```python
from build123d import *

# Parameters (mm, degrees)
CUT_EXTRUDE4_DEPTH      = 10.5250001
CUT_EXTRUDE4_DEPTH_BACK = 10.5250001
CHAMFER1_SIZE           = 0.762


with BuildPart() as part:
    # Sketch1 → Revolve1 (revolve)
    with BuildSketch(Plane(origin=(0, 0, 0), x_dir=(0, 0, -1), z_dir=(1, 0, 0))):
        with BuildLine():
            Line((0, 0), (3.175, 0))
            Line((3.175, 0), (3.175, 9.4996))
            Line((3.175, 9.4996), (9.525, 9.4996))
            Line((9.525, 9.4996), (9.525, 12.7))
            ThreePointArc((9.525, 12.7), (4.820045897, 13.835459863), (0, 14.2748))
            Line((0, 14.2748), (0, 0))
        make_face()
    revolve(axis=Axis((0, 0, 0), (0, 1, 0)))

    # Sketch2 → Cut-Extrude4 (cut, two sides)
    with BuildSketch(Plane(origin=(0, 0, 0), x_dir=(0, 0, -1), z_dir=(1, 0, 0))) as cut_extrude4_sk:
        Polygon((-0.7874, 59.433466129), (-0.7874, 14.251322907), (-0.7874, 11.8872), (0.7874, 11.8872), (0.7874, 14.251322907), (0.7874, 59.433466129), (0.7874, 149.797752573), (-0.7874, 149.797752573), align=None)
    extrude(amount=CUT_EXTRUDE4_DEPTH, mode=Mode.SUBTRACT)
    extrude(cut_extrude4_sk.sketch, amount=-CUT_EXTRUDE4_DEPTH_BACK, mode=Mode.SUBTRACT)

    # Chamfer1
    chamfer1_edges = [part.edges().sort_by_distance(p)[0] for p in [
        (0, 0, 3.175),
    ]]
    chamfer(chamfer1_edges, length=CHAMFER1_SIZE)


solid = part.part
```
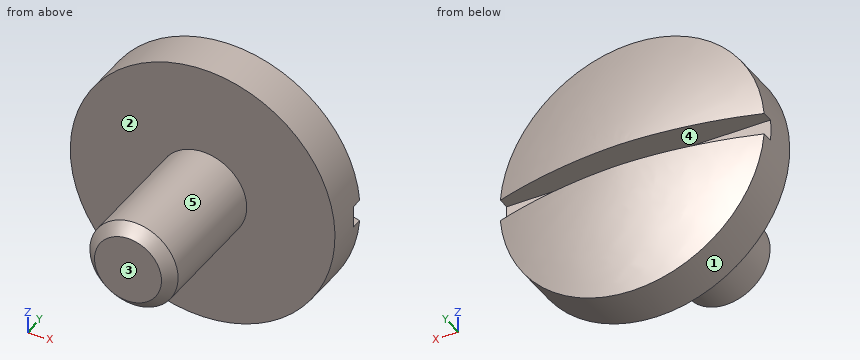
Source: CAD feature listing. Evaluate the final solid. Frame: model axes, mm. Face numbers are marked on the shaded views. A direction names the side the tool comes from. Coordinates: 2 decimals unless noted, no trailing zeros. Write each loop counter-clockwise with the first axis right and the second up, starting at its lowest first coordinate (ties: lowest second). Pieces come first, ordered by that corner, then holes. Notation, with made-up numbers: (34, 59) -> (85, 59) arc R19 ccw to (85, 65) -> close; hole circle Ø3 at (64, 26). An arc over 180 degrees is marked (long way). Return JSON: item names as keys, results as strings. Group by question number.
1) Mould query, pull axis Z, two halves, no side actions, for the marked faces 3, 4 and 5. Classes: +Z half, -Z half, draft (parallel to the pull), parting line (faces both ways), or undercut.
2) Set-up query: the marked faces 1 and 2. Return all of +Z, -Z, +X, -X, +Y, -Y with unobstructed straight access to the full face (end or side cutting, diameter ignored); none if empty.
3) Section query A-A, the plane z = 0. Return loops of the section in (x, y) (3 decimals).
4) Section query B-B, the plane y = 1.5. Return loops of the section in (x, z) (3 decimals), plus the area to 3 significant figures.
5) Contact query for flat-ended pins moving along their axis: P1, Ø8, axis at x = 0.5, z = 7.5, coming from the -Y side; P2, Ø8, axis at x = 3.5, y = 2.5, coming from the +Z side (3 decimals); P3, Ø6, axis at y = 12, z = -4.5, coming from the +X side; P4, Ø6, axis at x = 7.5, y = 2, coming from the -Z side. Output: stop coordinate, or through.
6) Ray query, line 1 along Y through (x, z) = (1.5, -0.5); line 2 along Z through (x, y) = (2.25, 12.25); line 3 along X through (y, z) = (12.5, 3.5). Return the intervals inside material, ascending.
From the geometry:
{
 "1": {"face 3": "draft", "face 4": "undercut", "face 5": "parting line"},
 "2": {"face 1": "+Y, -Y", "face 2": "-Y"},
 "3": {"outline": "(-9.525, 9.5) -> (-3.175, 9.5) -> (-3.175, 0.762) -> (-2.413, 0) -> (2.413, 0) -> (3.175, 0.762) -> (3.175, 9.5) -> (9.525, 9.5) -> (9.525, 11.887) -> (-9.525, 11.887) -> close"},
 "4": {"outline": "circle Ø6.35 at (0, 0)", "area": "31.7 mm²"},
 "5": {"P1": "y = 9.5", "P2": "z = 3.175", "P3": "x = 9.41", "P4": "through"},
 "6": {"line 1": "0 to 11.89", "line 2": "-9.26 to -0.79, 0.79 to 9.26", "line 3": "-8.86 to 8.86"}
}
